Work out the finished part from the listing and answer in its coordinate system (mm). Give positions to 0.01 mm unless a question says otherwise; leave off trailing zeros. Write each loop counter-clockwise with the first axis right and the second up, starting at its lowest first coordinate (ties: lowest second). Pieces come first, ordered by that corner, then holes. Notation, with made-up numbers: (27, 41) - (59, 41) arc R33 cw to (59, 75) - close; hole circle Ø2 at (12.5, -37). An arc over 180 degrees is marked (long way). Write item = value, one per line.
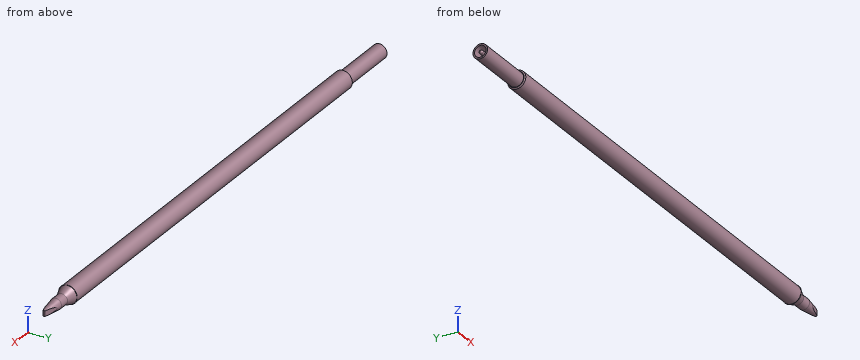
from build123d import *

# Parameters (mm, degrees)
FILLET1_R          = 0.45
CHAMFER1_SIZE      = 0.2
CHAMFER1_SIZE2     = 0.346410162
SKETCH2_R          = 0.05
CUT_EXTRUDE1_DEPTH = 5
FILLET3_R          = 0.1


with BuildPart() as part:
    # Sketch1 → Revolve1 (revolve)
    with BuildSketch(Plane.XY, mode=Mode.PRIVATE) as revolve1_sk:
        Polygon((0, 0), (-15, 0), (-15, 0.5), (0, 0.5), (0, 1.49), (-15, 1.49), (-15, 1.9), (0, 1.9), (0, 2.365), (115, 2.365), (117.5, 1.45), (120, 1.45), (125, 0.75), (125, 0), align=None)
    revolve(revolve1_sk.sketch.rotate(Axis((0, 0, 0), (1, 0, 0)), 90), axis=Axis((0, 0, 0), (1, 0, 0)))

    # Fillet1
    fillet1_edges = [part.edges().sort_by_distance(p)[0] for p in [
        (-15, 0, -0.5),
    ]]
    fillet(fillet1_edges, radius=FILLET1_R)

    # Chamfer1
    chamfer1_edges = [part.edges().sort_by_distance(p)[0] for p in [
        (0, 0, -2.365),
    ]]
    chamfer1_side = [part.faces().sort_by_distance(p)[0] for p in [
        (57.5, 0, -2.365),
    ]]
    chamfer(chamfer1_edges, length=CHAMFER1_SIZE, length2=CHAMFER1_SIZE2, reference=chamfer1_side[0])

    # Sketch2 → Revolve2 (revolve)
    with BuildSketch(Plane.XY, mode=Mode.PRIVATE) as revolve2_sk:
        with Locations((115, 2.365)):
            Circle(SKETCH2_R)
    revolve(revolve2_sk.sketch.rotate(Axis((0, 0, 0), (1, 0, 0)), 270), axis=Axis((0, 0, 0), (1, 0, 0)))

    # Sketch3 → Cut-Extrude1 (cut, symmetric)
    with BuildSketch(Plane.XY):
        Polygon((120, 1.65), (126, 0), (120, -1.65), (129.159329982, -1.65), (129.159329982, 1.65), align=None)
    extrude(amount=CUT_EXTRUDE1_DEPTH, both=True, mode=Mode.SUBTRACT)

    # Fillet3
    fillet3_edges = [part.edges().sort_by_distance(p)[0] for p in [
        (125, -0.275, 0),
        (125, 0.275, 0),
    ]]
    fillet(fillet3_edges, radius=FILLET3_R)


solid = part.part
1. Straight lines are drawn through the part: line 1 (Y direction, x = -11, z = 0); line 2 (Z direction, x = 56.5, y = -0.15); line 3 (Y direction, x = 64, z = -1.2). For each, find the intervals that lie inside material, in ascending order.
Solution:
line_1 = -1.9 to -1.49, -0.5 to 0.5, 1.49 to 1.9
line_2 = -2.36 to 2.36
line_3 = -2.04 to 2.04
2. Find section A-A, the plane x = 43. Give the vertices of the cut face in (y, z) (3 decimals).
Solution:
outline = circle Ø4.73 at (0, 0)
3. Given pin 1 (0.9 mm diameter, centred on y = -0.5, z = 0, fed in from -X); pin 2 (1 mm diameter, centred on x = 50.5, z = 1.5, fed in from -Y), each flat-ended and moving along its own axis, determine where each tip first touches the part or whether it passes through.
Solution:
pin_1 = -15
pin_2 = -2.14
